```python
from build123d import *

# Parameters (mm, degrees)
SKETCH2_R          = 0.8
CUT_EXTRUDE1_DEPTH = 3.5
CHAMFER1_SIZE      = 0.2
SKETCH3_R          = 1.25
CUT_EXTRUDE2_DEPTH = 4


with BuildPart() as part:
    # Sketch1 → Revolve1 (revolve)
    with BuildSketch(Plane(origin=(0, 0, 0), x_dir=(0, 0, -1), z_dir=(1, 0, 0))):
        with BuildLine():
            Line((0, 25.0571), (-4.944, 25.0571))
            Line((-4.944, 25.0571), (-4.944, 24.2951))
            Line((-4.944, 24.2951), (-5.680470391, 25.264317516))
            ThreePointArc((-5.680470391, 25.264317516), (-6.722, 25.781), (-7.763529609, 25.264317516))
            Line((-7.763529609, 25.264317516), (-8.5, 24.2951))
            Line((-8.5, 24.2951), (-8.5, 25.0571))
            Line((-8.5, 25.0571), (-12, 25.0571))
            Line((-12, 25.0571), (-12, 28.575))
            Line((-12, 28.575), (-18, 28.575))
            Line((-18, 28.575), (-18, 22.733))
            Line((-18, 22.733), (-17.3396, 22.733))
            Line((-17.3396, 22.733), (-17.975134466, 22.405795686))
            ThreePointArc((-17.975134466, 22.405795686), (-18.4572, 21.6154), (-17.975134466, 20.825004314))
            Line((-17.975134466, 20.825004314), (-17.3396, 20.4978))
            Line((-17.3396, 20.4978), (-18, 20.4978))
            Line((-18, 20.4978), (-18, 19.0571))
            Line((-18, 19.0571), (0, 19.0571))
            Line((0, 19.0571), (0, 25.0571))
        make_face()
    revolve(axis=Axis((0, 0, 0), (0, 0, 1)))

    # Sketch2 → Cut-Extrude1 (cut)
    with BuildSketch(Plane.XY.offset(18)):
        with Locations((-25.4, 0)):
            Circle(SKETCH2_R)
        with Locations((-12.7, 21.997045256)):
            Circle(SKETCH2_R)
        with Locations((12.7, 21.997045256)):
            Circle(SKETCH2_R)
        with Locations((25.4, 0)):
            Circle(SKETCH2_R)
        with Locations((12.7, -21.997045256)):
            Circle(SKETCH2_R)
        with Locations((-12.7, -21.997045256)):
            Circle(SKETCH2_R)
    extrude(amount=-CUT_EXTRUDE1_DEPTH, mode=Mode.SUBTRACT)

    # Chamfer1
    chamfer1_edges = [part.edges().sort_by_distance(p)[0] for p in [
        (0, -20.4978, 18),
        (0, -22.733, 18),
        (0, -25.0571, 8.5),
        (0, -25.0571, 4.944),
        (0, -25.0571, 0),
    ]]
    chamfer(chamfer1_edges, length=CHAMFER1_SIZE)

    # Sketch3 → Cut-Extrude2 (cut)
    with BuildSketch(Plane(origin=(0, 0, 0), x_dir=(-1, 0, 0), z_dir=(0, 0, -1))):
        with Locations((0, 21.5)):
            Circle(SKETCH3_R)
        with Locations((21.5, 0)):
            Circle(SKETCH3_R)
        with Locations((0, -21.5)):
            Circle(SKETCH3_R)
        with Locations((-21.5, 0)):
            Circle(SKETCH3_R)
    extrude(amount=-CUT_EXTRUDE2_DEPTH, mode=Mode.SUBTRACT)


solid = part.part
```
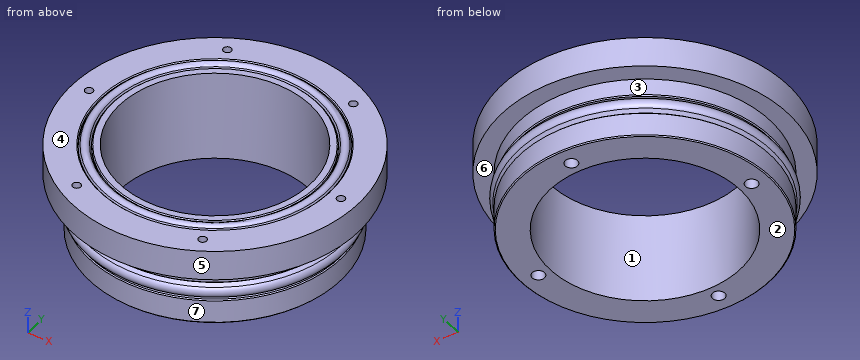
Geometry: final body of the model. Coordinates: model frame, mm. Face numbers are marked on the shaded views. A direction names the side the tool comes from. Round coordinates to 2 decimals unless told otherwise and drop trailing zeros. Write each loop counter-clockwise with the first axis right and the second up, starting at its lowest first coordinate (ties: lowest second). Pieces come first, ordered by that corner, then holes.
Item 1: Pin query (flat end, axial travel): P1, Ø2, axis at x = 25.4, y = 0, coming from the +Z side; P2, Ø2, axis at x = 5.5, z = 13.5, coming from the -Y side; P3, Ø4, axis at y = 8.5, z = 15, coming from the +X side; P4, Ø15, axis at x = -9, y = 7, coming from the -Z side. Return the tip coordinate at first contact, or that it passes through.
Item 2: Section query A-A (z = 15.75). Return loops of the section in (x, y) (3 decimals).
Item 3: Set-up query: the marked faces 4, 5, 6 and 7. Return all of +Z, -Z, +X, -X, +Y, -Y with unobstructed straight access to the full face (end or side cutting, diameter ignored); none if empty.
Item 4: Material intervals for L1, parallel to Y at x = 0, z = 2.25; L2, parallel to Y at x = -12.7, z = 16.75; L3, parallel to X at y = 11.5, z = 16.25, sorted ascending.
Item 5: Mould query, pull axis Z, two halves, no side actions, for the marked faces 1, 2 and 3. Classes: +Z half, -Z half, draft (parallel to the pull), parting line (faces both ways), or undercut.
Completed:
1. P1: stops at z = 18
1. P2: stops at y = -28.22
1. P3: stops at x = 27.83
1. P4: passes through
2. outline: circle Ø57.15 at (0, 0); hole circle Ø1.6 at (-25.4, 0); hole circle Ø38.114 at (0, 0); hole circle Ø1.6 at (-12.7, -21.997); hole circle Ø1.6 at (-12.7, 21.997); hole circle Ø1.6 at (12.7, -21.997); hole circle Ø1.6 at (12.7, 21.997); hole circle Ø1.6 at (25.4, 0)
3. face 4: +Z
3. face 5: +Z, -Z
3. face 6: none
3. face 7: -Z
4. L1: y = -25.06 to -22.75, -20.25 to -19.06, 19.06 to 20.25, 22.75 to 25.06
4. L2: y = -25.6 to -22.8, -21.2 to -14.21, 14.21 to 21.2, 22.8 to 25.6
4. L3: x = -26.16 to -15.2, 15.2 to 26.16
5. face 1: draft
5. face 2: -Z half
5. face 3: undercut
